Design review of the part built by this model. Coordinates are the model's own, in mm. Face numbers are marked on the shaded views. A direction names the side the tool comes from. Round coordinates to 2 decimals unless told otherwise and drop trailing zeros. Write each loop counter-clockwise with the first axis right and the second up, starting at its lowest first coordinate (ties: lowest second). Pieces come first, ordered by that corner, then holes. Notation, with made-up numbers: (6, 44.25) -> (46, 44.25) arc R12 ccw to (46, 63.25) -> close; hole circle Ø3 at (69.5, 45). An arc over 180 degrees is marked (long way). One line per question, with ' | ' between items. Start each with the question number.
1) Consider section B-B (z = 25). Give the boundary of the cut face in (x, y).
2) For the marked faces 4, 5 and 6, list the 3-axis set-ups (+Z, -Z, +X, -X, +Y, -Y) from which the entire face can be reached by the end or side of a thin tool; tool diameter is ignored.
3) For probe 1 along Z at (x, y) = (-21, -1); probe 2 along Z at (x, y) = (12.5, -17.5); probe 3 along X at (y, z) = (-5.5, 44.5), list the stretches that pass through material, from the lowest coordinate up.
4) Mouldability with a two-part tool opening along Z and no side actions: class the marked faces 1, 2 and 3 as +Z half, -Z half, draft (parallel to the pull), parting line (faces both ways), or undercut.
5) Consider section A-A (x = -15). Give the boundary of the cut face in (y, z), then the cut area to 3 significant figures.
6) Consider section D-D (z = 43.5). Give the boundary of the cut face in (x, y).
7) Consider section C-C (x = 28). Give the boundary of the cut face in (y, z), then the cut area to 3 significant figures.
8) Insertion check: pin 1 Ø2 at (y, z) = (-6, 38) entering from +X; pin 2 Ø4 at (x, y) = (6, 15) entering from +Z; pin 3 Ø25 at (x, y) = (14.5, 0.5) entering from -Z; pin 4 Ø12 at (x, y) = (-11.5, -9) entering from -Z. Each pin has a flat end and moves straight along its axis. Give the tip position at first contact, or say it passes through.
```python
from build123d import *

# Parameters (mm, degrees)
SKETCH1_R               = 11
BOSS_EXTRUDE1_DEPTH     = 50
SKETCH2_R               = 17.5
CUT_EXTRUDE1_DEPTH      = 2
SKETCH3_R               = 10
CUT_EXTRUDE2_DEPTH      = 109.696290771
CUT_EXTRUDE3_DEPTH      = 75.521428374
CUT_EXTRUDE3_DEPTH_BACK = 4
SKETCH4_R               = 11
CUT_EXTRUDE4_DEPTH      = 75.521428307
CUT_EXTRUDE4_DEPTH_BACK = 4
SKETCH5_R               = 11
SKETCH6_W               = 90
SKETCH6_H               = 30
CUT_EXTRUDE5_DEPTH      = 86.950914215
SKETCH7_R               = 2.5
CUT_EXTRUDE6_DEPTH      = 75.521428207
FILLET2_R               = 5


with BuildPart() as part:
    # Sketch1 → Boss-Extrude1 (new body)
    with BuildSketch(Plane.XY):
        with BuildLine():
            Line((35.445784896, -24.19527897), (-46.137339056, -24.19527897))
            Line((-46.137339056, -24.19527897), (-46.137339056, 25.80472103))
            Line((-46.137339056, 25.80472103), (35.445784896, 25.80472103))
            ThreePointArc((35.445784896, 25.80472103), (48.862660944, 0.80472103), (35.445784896, -24.19527897))
        make_face()
        with Locations((18.862660944, 0.80472103)):
            Circle(SKETCH1_R, mode=Mode.SUBTRACT)
    extrude(amount=BOSS_EXTRUDE1_DEPTH)

    # Sketch2 → Cut-Extrude1 (cut)
    with BuildSketch(Plane.ZY.offset(46.137339056)):
        with Locations((25, 0.80472103)):
            Circle(SKETCH2_R)
    extrude(amount=-CUT_EXTRUDE1_DEPTH, mode=Mode.SUBTRACT)

    # Sketch3 → Cut-Extrude2 (cut, through all)
    with BuildSketch(Plane.ZY.offset(44.137339056)):
        with Locations((25, 0.80472103)):
            Circle(SKETCH3_R)
    extrude(amount=-CUT_EXTRUDE2_DEPTH, mode=Mode.SUBTRACT)

    # Sketch4 → Cut-Extrude3 (cut, two sides: drawn at the far end of the back side and taken through both)
    with BuildSketch(Plane.XY.offset(50).offset(-CUT_EXTRUDE3_DEPTH_BACK)):
        with BuildLine():
            Line((35.445784896, 25.80472103), (-20.137339056, 25.80472103))
            Line((-20.137339056, 25.80472103), (-1.938827342, -24.19527897))
            Line((-1.938827342, -24.19527897), (35.445784896, -24.19527897))
            ThreePointArc((35.445784896, -24.19527897), (48.862660944, 0.80472103), (35.445784896, 25.80472103))
        make_face()
        with Locations((18.862660944, 0.80472103)):
            Circle(SKETCH4_R, mode=Mode.SUBTRACT)
    extrude(amount=CUT_EXTRUDE3_DEPTH + CUT_EXTRUDE3_DEPTH_BACK, mode=Mode.SUBTRACT)

    # Sketch5 → Cut-Extrude4 (cut, two sides: drawn at the far end of the back side and taken through both)
    with BuildSketch(Plane(origin=(0, 0, 0), x_dir=(-1, 0, 0), z_dir=(0, 0, -1)).offset(-CUT_EXTRUDE4_DEPTH_BACK)):
        with BuildLine():
            Line((1.938827342, -24.19527897), (20.137339056, 25.80472103))
            Line((20.137339056, 25.80472103), (-35.445784896, 25.80472103))
            ThreePointArc((-35.445784896, 25.80472103), (-48.862660944, 0.80472103), (-35.445784896, -24.19527897))
            Line((-35.445784896, -24.19527897), (1.938827342, -24.19527897))
        make_face()
        with Locations((-18.862660944, 0.80472103)):
            Circle(SKETCH5_R, mode=Mode.SUBTRACT)
    extrude(amount=CUT_EXTRUDE4_DEPTH + CUT_EXTRUDE4_DEPTH_BACK, mode=Mode.SUBTRACT)

    # Sketch6 → Cut-Extrude5 (cut, through all)
    with BuildSketch(Plane(origin=(0, 25.80472103, 0), x_dir=(1, 0, 0), z_dir=(0, 1, 0))):
        with Locations((13.862660944, -25)):
            Rectangle(SKETCH6_W, SKETCH6_H)
    extrude(amount=-CUT_EXTRUDE5_DEPTH, mode=Mode.SUBTRACT)

    # Sketch7 → Cut-Extrude6 (cut, through all)
    with BuildSketch(Plane.XY.offset(50)):
        with Locations((-21.137339056, -7.19527897)):
            Circle(SKETCH7_R)
    extrude(amount=-CUT_EXTRUDE6_DEPTH, mode=Mode.SUBTRACT)

    # Fillet2
    fillet2_edges = [part.edges().sort_by_distance(p)[0] for p in [
        (-31.137339056, 0.80472103, 10),
        (-31.137339056, 0.80472103, 40),
    ]]
    fillet(fillet2_edges, radius=FILLET2_R - 0.0001)  # a hair under: the kernel refuses the full size


solid = part.part
```
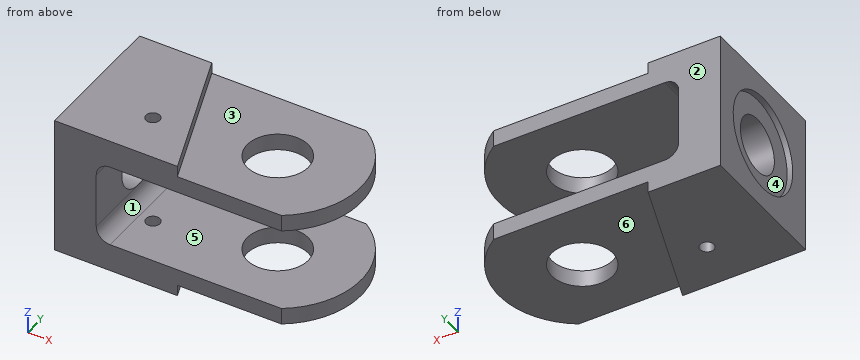
From the geometry:
1) outline: (-46.14, -24.2) -> (-31.14, -24.2) -> (-31.14, -9.2) -> (-44.14, -9.2) -> (-44.14, -16.7) -> (-46.14, -16.7) -> close; (-46.14, 18.3) -> (-44.14, 18.3) -> (-44.14, 10.8) -> (-31.14, 10.8) -> (-31.14, 25.8) -> (-46.14, 25.8) -> close
2) face 4: -X | face 5: +X, +Y, -Y | face 6: -Z, +X, +Y
3) probe 1: z = 0 to 10, 40 to 50 | probe 2: z = 4 to 10, 40 to 46 | probe 3: x = -46.14 to -22.97, -19.3 to 9.85, 27.88 to 48.19
4) face 1: undercut | face 2: draft | face 3: +Z half
5) outline: (-24.2, 0) -> (11.69, 0) -> (11.69, 4) -> (25.8, 4) -> (25.8, 10) -> (-24.2, 10) -> close; (-24.2, 40) -> (25.8, 40) -> (25.8, 46) -> (11.69, 46) -> (11.69, 50) -> (-24.2, 50) -> close | area: 887 mm2
6) outline: (-46.14, -24.2) -> (35.45, -24.2) arc R30 ccw to (35.45, 25.8) -> (-46.14, 25.8) -> close; hole circle Ø5 at (-21.14, -7.2); hole circle Ø22 at (18.86, 0.8)
7) outline: (-24.2, 4) -> (-5.32, 4) -> (-5.32, 10) -> (-24.2, 10) -> close; (-24.2, 40) -> (-5.32, 40) -> (-5.32, 46) -> (-24.2, 46) -> close; (6.93, 4) -> (25.8, 4) -> (25.8, 10) -> (6.93, 10) -> close; (6.93, 40) -> (25.8, 40) -> (25.8, 46) -> (6.93, 46) -> close | area: 453 mm2
8) pin 1: stops at x = -29.14 | pin 2: stops at z = 46 | pin 3: stops at z = 4 | pin 4: stops at z = 0
